CAD build for the part. Positions are in the model's coordinates, mm. Face numbers are marked on the shaded views. Coordinates: 2 decimals unless noted, no trailing zeros. Loops run counter-clockwise (first coordinate to the right, second up) from the corner with the lowest first, then second, coordinate; pieces in that order, holes last.
1) Pin check, flat tips, straight feed: pin 1 Ø1.4 at (x, y) = (-5.5, 2) entering from +Z; pin 2 Ø2 at (x, y) = (2, -2) entering from +Z; pin 3 Ø0.9 at (x, y) = (5.5, -1) entering from +Z; pin 4 Ø2 at (y, z) = (-9, -0.5) entering from +X. Stop position of each tip, or through.
2) Two-plate mould, pull along X, no slides. Class the marked faces 1, 2, 3 and 4: +X half, -X half, draft (parallel to the pull), parting line (faces both ways), or undercut.
3) Wall check: line 1 along X through (y, z) = (0, 1); line 2 along Y through (x, z) = (-1, 0.25). Give the ranges that are in metal, low to high.
4) Saw through at B-B, the plane y = 0. Write the cut outline in (x, z), and give its area (3 significant figures).
5) Saw through at D-D, the plane x = 8. Write the cut outline in (y, z).
6) Saw through at C-C, the plane z = 4.25. Write the cut outline in (x, y).
7) Saw through at A-A, the plane x = 0. Write the cut outline in (y, z).
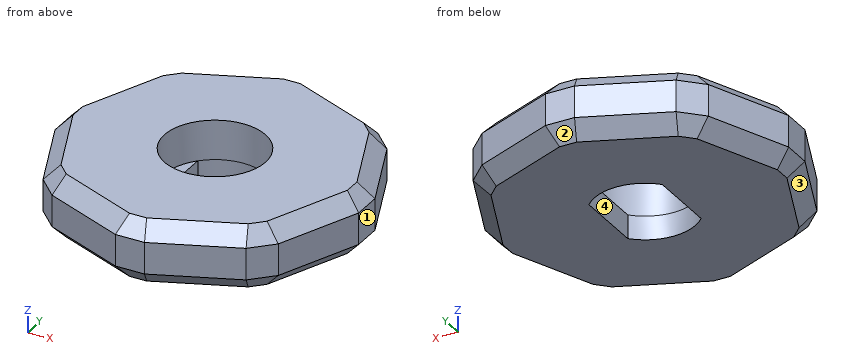
```python
from build123d import *

# Parameters (mm, degrees)
PAD_DEPTH      = 5
PAD_DEPTH_BACK = 3
SKETCH002_R    = 6.4
POCKET_DEPTH   = 5.001
CHAMFER_SIZE   = 2


with BuildPart() as part:
    # Sketch → Pad (new body, two sides)
    with BuildSketch(Plane.XY) as pad_sk:
        Polygon((0, 20), (-14.142136, 14.142136), (-20, 0), (-14.142136, -14.142136), (0, -20), (14.142136, -14.142136), (20, 0), (14.142136, 14.142136), align=None)
        with BuildLine():
            Line((4.65, 4.397442), (4.65, -4.397442))
            ThreePointArc((-4.65, -4.397442), (0, -6.4), (4.65, -4.397442))
            Line((-4.65, 4.397442), (-4.65, -4.397442))
            ThreePointArc((4.65, 4.397442), (0, 6.4), (-4.65, 4.397442))
        make_face(mode=Mode.SUBTRACT)
    extrude(amount=PAD_DEPTH)
    extrude(pad_sk.sketch, amount=-PAD_DEPTH_BACK)

    # Sketch002 → Pocket (cut, through all)
    with BuildSketch(Plane.XY):
        Circle(SKETCH002_R)
    extrude(amount=POCKET_DEPTH, mode=Mode.SUBTRACT)

    # Chamfer
    chamfer_edges = [part.edges().sort_by_distance(p)[0] for p in [
        (0, -20, 1),
        (14.142136, -14.142136, 1),
        (7.071068, -17.071068, -3),
        (7.071068, -17.071068, 5),
        (-14.142136, -14.142136, 1),
        (-7.071068, -17.071068, -3),
        (-7.071068, -17.071068, 5),
        (-20, 0, 1),
        (-17.071068, -7.071068, -3),
        (-17.071068, -7.071068, 5),
        (-14.142136, 14.142136, 1),
        (-17.071068, 7.071068, -3),
        (-17.071068, 7.071068, 5),
        (0, 20, 1),
        (-7.071068, 17.071068, -3),
        (-7.071068, 17.071068, 5),
        (14.142136, 14.142136, 1),
        (7.071068, 17.071068, -3),
        (7.071068, 17.071068, 5),
        (20, 0, 1),
        (17.071068, 7.071068, -3),
        (17.071068, 7.071068, 5),
        (17.071068, -7.071068, -3),
        (17.071068, -7.071068, 5),
    ]]
    chamfer(chamfer_edges, length=CHAMFER_SIZE)


solid = part.part
```
Data:
1. pin 1: stops at z = 5
1. pin 2: passes through
1. pin 3: stops at z = 0
1. pin 4: stops at x = 16.69
2. face 1: +X half
2. face 2: draft
2. face 3: -X half
2. face 4: undercut
3. line 1: x = -19.23 to -6.4, 6.4 to 19.23
3. line 2: y = -19.23 to -6.32, 6.32 to 19.23
4. outline: (-19.23, -1) - (-17.39, -3) - (-4.65, -3) - (-4.65, 0) - (-6.4, 0) - (-6.4, 5) - (-17.39, 5) - (-19.23, 3) - close; (4.65, -3) - (17.39, -3) - (19.23, -1) - (19.23, 3) - (17.39, 5) - (6.4, 5) - (6.4, 0) - (4.65, 0) - close
4. area: 208 mm2
5. outline: (-16.69, -1) - (-14.52, -3) - (14.52, -3) - (16.69, -1) - (16.69, 3) - (14.52, 5) - (-14.52, 5) - (-16.69, 3) - close
6. outline: (-18.08, -1.37) - (-13.75, -11.82) - (-11.82, -13.75) - (-1.37, -18.08) - (1.37, -18.08) - (11.82, -13.75) - (13.75, -11.82) - (18.08, -1.37) - (18.08, 1.37) - (13.75, 11.82) - (11.82, 13.75) - (1.37, 18.08) - (-1.37, 18.08) - (-11.82, 13.75) - (-13.75, 11.82) - (-18.08, 1.37) - close; hole circle Ø12.8 at (0, 0)
7. outline: (-19.23, -1) - (-17.39, -3) - (-6.4, -3) - (-6.4, 5) - (-17.39, 5) - (-19.23, 3) - close; (6.4, -3) - (17.39, -3) - (19.23, -1) - (19.23, 3) - (17.39, 5) - (6.4, 5) - close
